```python
from build123d import *

# Parameters (mm, degrees)
F0_R      = 3.175
F1_DEPTH  = 15.875
F3_R      = 6.35
F4_DEPTH  = 0.508
F1_FACE_R = 3.175


with BuildPart() as f1:
    # F0 (on Top) → F1 (new body)
    with BuildSketch(Plane.XY):
        Circle(F0_R)
    extrude(amount=F1_DEPTH)

    # F3 (on offset) → F4 (join)
    with BuildSketch(Plane.XY.offset(6.35)):
        Circle(F3_R)
    extrude(amount=F4_DEPTH)

    # F1_face (on face) → F7 section 0
    with BuildSketch(Plane.XY.offset(15.875), mode=Mode.PRIVATE) as f7_s0:
        Circle(F1_FACE_R)
    loft([f7_s0.sketch, Vertex(0, 0, 20.955)])


solid = f1.part
```
Work out the finished part from the listing and answer in its coordinate system (mm). A direction names the side the tool comes from. Give positions to 0.01 mm unless a question says otherwise; leave off trailing zeros. Write each loop counter-clockwise with the first axis right and the second up, starting at its lowest first coordinate (ties: lowest second). Pieces come first, ordered by that corner, then holes. Notation, with made-up numbers: (-21.75, 51) - (-11.75, 51) arc R13 ccw to (-11.75, 58) - close; hole circle Ø5 at (71, -25). An arc over 180 degrees is marked (long way). Use one line per item in the form item = value.
1. A cutting plane is placed at C-C (z = 19.75). Write down the section's boundary in (x, y), and give its area (3 significant figures).
Filled in:
outline = circle Ø1.51 at (0, 0)
area = 1.78 mm^2
2. A cutting plane is placed at B-B (x = 5). Write down the section's boundary in (y, z).
Filled in:
outline = (-3.91, 6.35) - (3.91, 6.35) - (3.91, 6.86) - (-3.91, 6.86) - close
3. For faces 1 (the face through (-2, 3, 6.858)), 2 (the face through (-0.69, -3.1, 3.13)), 3 (the face through (-1.38, -6.2, 6.6)), determine the directions among +Z, -Z, +X, -X, +Y, -Y from which every point of the face is accessible in a straight line to the end or side of a thin tool.
Filled in:
face_1 = +Z
face_2 = -Z
face_3 = +Z, -Z
4. Each of these flat-tipped pins is pushed along its axis until it touches: pin 1 Ø4 at (y, z) = (1.5, 9) entering from +X (3 decimals); pin 2 Ø3 at (x, y) = (4.5, -3.5) entering from -Z; pin 3 Ø1.5 at (x, z) = (5, 7) entering from +Y; pin 4 Ø6.5 at (x, y) = (-2, -1.5) entering from +Z (3 decimals). Where does it stop, or does it pass through?
Filled in:
pin_1 = 3.175
pin_2 = 6.35
pin_3 = 4.71
pin_4 = 20.955
5. A cutting plane is placed at A-A (z = 12). Write down the section's boundary in (x, y) (3 decimals), and give its area (3 significant figures).
Filled in:
outline = circle Ø6.35 at (0, 0)
area = 31.7 mm^2
6. A cutting plane is placed at D-D (x = -3.5). Write down the section's boundary in (y, z), and give its area (3 significant figures).
Filled in:
outline = (-5.3, 6.35) - (5.3, 6.35) - (5.3, 6.86) - (-5.3, 6.86) - close
area = 5.38 mm^2
7. Consider L1, parallel to Z at x = -3.5, y = 2.5; L2, parallel to X at y = 0, z = 5.5 (3 decimals); L3, parallel to Y at x = 0.25, z = 3.75. Determine where each line is inside the solid, lowest interval first.
Filled in:
L1 = 6.35 to 6.86
L2 = -3.175 to 3.175
L3 = -3.17 to 3.17
